Build history of the part. All positions in model axes, mm. A direction names the side the tool comes from. Round coordinates to 2 decimals unless told otherwise and drop trailing zeros. Loops run counter-clockwise (first coordinate to the right, second up) from the corner with the lowest first, then second, coordinate; pieces in that order, holes last. Notation, with made-up numbers: (-22.5, 3) - (33.5, 3) arc R21 cw to (33.5, 39) - close; hole circle Ø6 at (12, -25.75). An arc over 180 degrees is marked (long way). Use one line per item in the form item = value. Start each with the question number.
Q1. Saw through at A-A (x = -67). Give the cut face in (y, z).
Q2. 3-axis set-ups, long thin cutter, end or side, ignore diameter. For faces 1 (the face through (3, 87, -25)), 2 (the face through (45, -30, 6)), 3 (the face through (-51.203, 8.743, 1.098)), 4 (the face through (98, 67, -10)), 5 (the face through (97.605, 72.454, -9.8)): which of +Z, -Z, +X, -X, +Y, -Y reach the whole face in a straight line?
Q3. Saw through at B-B (y = -77). Give the cut face in (x, z).
Q4. Saw through at C-C (x = 33.5). Give the cut face in (y, z).
Q5. Pin check, flat tips, straight feed: pin 1 (2.5 mm diameter, centred on y = -19, z = 6, fed in from +X); pin 2 (6.5 mm diameter, centred on y = 45.5, z = -1.5, fed in from +X); pin 3 (8 mm diameter, centred on x = -7, y = 27, fed in from +Z); pin 4 (7.5 mm diameter, centred on x = 99, y = 81, fed in from -Z). Stop position of each tip, or through.
Q6. Drill centre lines: line 1 (Y direction, x = -37, z = 5); line 2 (X direction, y = 47, z = 2.75); line 3 (X direction, y = -67, z = -2.5). Where is each one in solid material? Low to high.
Q7. Saw through at D-D (y = 29). Give the cut face in (x, z).
Q8. Mould opens along Y. For faces 6 (the face through (-1, -95, -21)), 7 (the face through (1, 95, -21)), 8 (the face through (3, -18, 0)) say: released by +Y, released by -Y, zero draft, split by the parting line, or undercut.
```python
from build123d import *

# Parameters (mm, degrees)
SKETCH_1_W               = 210
SKETCH_1_H               = 190
EXTRUDE_1_DEPTH          = 8
EXTRUDE_2_DEPTH          = 50
SKETCH_3_W               = 20
SKETCH_3_H               = 20
EXTRUDE_3_DEPTH          = 15
SKETCH_8_R               = 4.55
CUT_EXTRUDE_1_DEPTH      = 25
SKETCH_9_W               = 120
SKETCH_9_H               = 100
EXTRUDE_4_DEPTH          = 12
SKETCH_10_R              = 15
CUT_EXTRUDE_2_DEPTH      = 147.608321728
SKETCH_13_R              = 4.55
CUT_EXTRUDE_3_DEPTH      = 154.016338997
PATTERN_CIRCULAR_2_COUNT = 4
SKETCH_14_W              = 120
SKETCH_14_H              = 100
CUT_EXTRUDE_4_DEPTH      = 6
SKETCH_15_R              = 1.85
CUT_EXTRUDE_5_DEPTH      = 10
SKETCH_16_W              = 68
SKETCH_16_H              = 76
EXTRUDE_5_DEPTH          = 13
SKETCH_17_W              = 60
SKETCH_17_H              = 60
CUT_EXTRUDE_6_DEPTH      = 5


with BuildPart() as part:
    # 스케치1 → 보스-돌출1 (new body)
    with BuildSketch(Plane.XY):
        Rectangle(SKETCH_1_W, SKETCH_1_H)
    extrude(amount=EXTRUDE_1_DEPTH)

    # 스케치2 → 보스-돌출2 (add)
    with BuildSketch(Plane(origin=(0, 0, 0), x_dir=(-1, 0, 0), z_dir=(0, 0, -1))):
        Polygon((-105, 95), (105, 95), (105, -95), (-105, -95), (-105, -87), (97, -87), (97, 87), (-105, 87), align=None)
    extrude(amount=EXTRUDE_2_DEPTH)

    # 스케치3 → 보스-돌출3 (add)
    with BuildSketch(Plane(origin=(105, 0, 0), x_dir=(0, 0, -1), z_dir=(1, 0, 0))):
        with Locations((10, 77)):
            Rectangle(SKETCH_3_W, SKETCH_3_H)
    extrude_3 = extrude(amount=-EXTRUDE_3_DEPTH)

    # 스케치8 → 컷-돌출1 (cut)
    with BuildSketch(Plane(origin=(105, 0, 0), x_dir=(0, 0, -1), z_dir=(1, 0, 0))):
        with Locations(Location((10, 77, 0), (0, 0, 90))):
            Circle(SKETCH_8_R)
    cut_extrude_1 = extrude(amount=-CUT_EXTRUDE_1_DEPTH, mode=Mode.SUBTRACT)

    # 대칭 복사1: 보스-돌출3, 컷-돌출1 across plane
    add(extrude_3.mirror(Plane(origin=(0, 0, 0), x_dir=(0, 0, 1), z_dir=(0, -1, 0))))
    add(cut_extrude_1.mirror(Plane(origin=(0, 0, 0), x_dir=(0, 0, 1), z_dir=(0, -1, 0))), mode=Mode.SUBTRACT)

    # 스케치9 → 보스-돌출4 (add)
    with BuildSketch(Plane(origin=(0, 0, 0), x_dir=(-1, 0, 0), z_dir=(0, 0, -1))):
        with Locations((37, 37)):
            Rectangle(SKETCH_9_W, SKETCH_9_H)
    extrude(amount=EXTRUDE_4_DEPTH)

    # 스케치10 → 컷-돌출2 (cut, through all)
    with BuildSketch(Plane(origin=(0, 0, -12), x_dir=(-1, 0, 0), z_dir=(0, 0, -1))):
        with Locations((37, 37)):
            Circle(SKETCH_10_R)
    extrude(amount=-CUT_EXTRUDE_2_DEPTH, mode=Mode.SUBTRACT)

    # 스케치13 → 컷-돌출3 (cut, through all)
    with BuildSketch(Plane.XY.offset(8)):
        with Locations((-47, 67)):
            Circle(SKETCH_13_R)
        with Locations((-27, 67)):
            Circle(SKETCH_13_R)
    cut_extrude_3 = extrude(amount=-CUT_EXTRUDE_3_DEPTH, mode=Mode.SUBTRACT)

    # 원형 패턴2: 컷-돌출3 ×4 about axis
    pattern_circular_2_axis = Axis((-37, 37, 0), (0, 0, 1))
    for i in range(1, PATTERN_CIRCULAR_2_COUNT):
        add(cut_extrude_3.rotate(pattern_circular_2_axis, i * 360 / PATTERN_CIRCULAR_2_COUNT), mode=Mode.SUBTRACT)

    # 스케치14 → 컷-돌출4 (cut)
    with BuildSketch(Plane(origin=(0, 0, -12), x_dir=(-1, 0, 0), z_dir=(0, 0, -1))):
        with Locations((37, 37)):
            Rectangle(SKETCH_14_W, SKETCH_14_H)
    extrude(amount=-CUT_EXTRUDE_4_DEPTH, mode=Mode.SUBTRACT)

    # 스케치15 → 컷-돌출5 (cut)
    with BuildSketch(Plane.XY.offset(8)):
        with Locations((-37, -45)):
            Circle(SKETCH_15_R)
        with Locations((-37, -15)):
            Circle(SKETCH_15_R)
    extrude(amount=-CUT_EXTRUDE_5_DEPTH, mode=Mode.SUBTRACT)

    # 스케치16 → 보스-돌출5 (add)
    with BuildSketch(Plane.XY.offset(8)):
        with Locations((71, -30)):
            Rectangle(SKETCH_16_W, SKETCH_16_H)
    extrude(amount=-EXTRUDE_5_DEPTH)

    # 스케치17 → 컷-돌출6 (cut)
    with BuildSketch(Plane.XY.offset(8)):
        with Locations((75, -30)):
            Rectangle(SKETCH_17_W, SKETCH_17_H)
    extrude(amount=-CUT_EXTRUDE_6_DEPTH, mode=Mode.SUBTRACT)


solid = part.part
```
Report:
q1.outline = (-95, -50) - (-87, -50) - (-87, 0) - (-13, 0) - (-13, -6) - (22.45, -6) - (22.45, 8) - (-95, 8) - close; (31.55, -6) - (42.45, -6) - (42.45, 8) - (31.55, 8) - close; (51.55, -6) - (87, -6) - (87, -50) - (95, -50) - (95, 8) - (51.55, 8) - close
q2.face_1 = -Z
q2.face_2 = +Z, +X
q2.face_3 = +Z, -Z
q2.face_4 = -Z, +X
q2.face_5 = +X
q3.outline = (-105, -50) - (-97, -50) - (-97, 0) - (90, 0) - (90, -5.45) - (105, -5.45) - (105, 8) - (-105, 8) - close; (90, -20) - (105, -20) - (105, -14.55) - (90, -14.55) - close
q4.outline = (-95, -50) - (-87, -50) - (-87, 0) - (87, 0) - (87, -50) - (95, -50) - (95, 8) - (-95, 8) - close
q5.pin_1 = 45
q5.pin_2 = 105
q5.pin_3 = through
q5.pin_4 = -20
q6.line_1 = -95 to -46.85, -43.15 to -16.85, -13.15 to 22, 52 to 95
q6.line_2 = -105 to -71.55, -62.45 to -48.18, -25.82 to -11.55, -2.45 to 105
q6.line_3 = -105 to -97, 37 to 105
q7.outline = (-105, -50) - (-97, -50) - (-97, -6) - (-71.09, -6) - (-71.09, 8) - (-105, 8) - close; (-62.91, -6) - (-49.69, -6) - (-49.69, 8) - (-62.91, 8) - close; (-24.31, -6) - (-11.09, -6) - (-11.09, 8) - (-24.31, 8) - close; (-2.91, -6) - (23, -6) - (23, 0) - (105, 0) - (105, 8) - (-2.91, 8) - close
q8.face_6 = released by -Y
q8.face_7 = released by +Y
q8.face_8 = undercut
